Build history of the part. All positions in model axes, mm. A direction names the side the tool comes from. Give positions to 0.01 mm unless a question says otherwise; leave off trailing zeros. Loops run counter-clockwise (first coordinate to the right, second up) from the corner with the lowest first, then second, coordinate; pieces in that order, holes last. Notation, with made-up numbers: M 54,31 L 105,31 A21 cw 105,47 Z; hole C -3.75,-21.75 d2. An arc over 180 degrees is marked long. Put each result on its own line as item: value.
```python
from build123d import *

# Parameters (mm, degrees)
SKETCH1_R               = 5
BOSS_EXTRUDE1_DEPTH     = 2
SKETCH4_R               = 3.9
BOSS_EXTRUDE2_DEPTH     = 16
CUT_EXTRUDE4_DEPTH      = 3
SKETCH3_5_R             = 1.7
CUT_EXTRUDE5_DEPTH      = 3
CUT_EXTRUDE5_DEPTH_BACK = 3.5
SKETCH5_W               = 6.581793069
SKETCH5_H               = 3
CUT_EXTRUDE6_DEPTH      = 6.0375


with BuildPart() as part:
    # Sketch1 → Boss-Extrude1 (new body)
    with BuildSketch(Plane(origin=(0, 0, 0), x_dir=(1, 0, 0), z_dir=(0, 1, 0))):
        Circle(SKETCH1_R)
    extrude(amount=BOSS_EXTRUDE1_DEPTH)

    # Sketch4 → Boss-Extrude2 (add)
    with BuildSketch(Plane(origin=(0, 0, 0), x_dir=(-1, 0, 0), z_dir=(0, -1, 0))):
        Circle(SKETCH4_R)
    extrude(amount=BOSS_EXTRUDE2_DEPTH)

    # Sketch3 → Cut-Extrude4 (cut)
    with BuildSketch(Plane(origin=(0, -13.5, 0), x_dir=(1, 0, 0), z_dir=(0, 1, 0))):
        Polygon((3.225944629, -0.0375), (1.580496362, 2.8125), (-1.710400172, 2.8125), (-3.35584844, -0.0375), (-1.710400172, -2.8875), (1.580496362, -2.8875), align=None)
    extrude(amount=CUT_EXTRUDE4_DEPTH, mode=Mode.SUBTRACT)

    # Sketch3<5> → Cut-Extrude5 (cut, two sides)
    with BuildSketch(Plane(origin=(0, -13.5, 0), x_dir=(1, 0, 0), z_dir=(0, 1, 0))) as cut_extrude5_sk:
        with Locations((-0.064951905, -0.0375)):
            Circle(SKETCH3_5_R)
    extrude(amount=CUT_EXTRUDE5_DEPTH, mode=Mode.SUBTRACT)
    extrude(cut_extrude5_sk.sketch, amount=-CUT_EXTRUDE5_DEPTH_BACK, mode=Mode.SUBTRACT)

    # Sketch5 → Cut-Extrude6 (cut, through all)
    with BuildSketch(Plane.XY.offset(0.0375)):
        with Locations((-0.064951906, -12)):
            Rectangle(SKETCH5_W, SKETCH5_H)
    extrude(amount=-CUT_EXTRUDE6_DEPTH, mode=Mode.SUBTRACT)


solid = part.part
```
Q1. Slice it at A-A (x = 1.25). List the corners of the cut face in (y, z).
Here are the results:
outline: M -16,-3.69 L -13.5,-3.69 L -13.5,-1.04 L -16,-1.04 Z; M -16,1.11 L -13.5,1.11 L -13.5,2.89 L -10.5,2.89 L -10.5,-3.69 L 0,-3.69 L 0,-4.84 L 2,-4.84 L 2,4.84 L 0,4.84 L 0,3.69 L -16,3.69 Z
Q2. Slice it at C-C (y = -11.75). List the corners of the cut face in (x, z).
Here are the results:
outline: M -3.36,-1.99 L -3.36,0.04 L -1.71,2.89 L 1.58,2.89 L 3.23,0.04 L 3.23,-2.19 A3.9 ccw long Z
Q3. Slice it at B-B (z = 2). List the corners of the cut face in (x, y).
Here are the results:
outline: M -4.58,0 L -3.35,0 L -3.35,-16 L 3.35,-16 L 3.35,0 L 4.58,0 L 4.58,2 L -4.58,2 Z; hole M -2.22,-13.5 L 2.09,-13.5 L 2.09,-10.5 L -2.22,-10.5 Z
Q4. Probe line 1 (Y direction, x = 1.5, z = -1.75); line 2 (X direction, y = -14.75, z = 0); line 3 (Y direction, x = -1.25, z = -4.5). List the from-to ranges inside material, lowest first. Write a range as from..to.
Here are the results:
line 1: -16..-13.5, -10.5..2
line 2: -3.9..-1.76, 1.63..3.9
line 3: 0..2
Q5. Slice it at D-D (y = -13.75). List the corners of the cut face in (x, z), and give its area (3 significant figures).
Here are the results:
outline: C 0,0 d7.8; hole C -0.06,0.04 d3.4
area: 38.7 mm²
Q6. Tool access for faces 4 (the flat face through (0, 2, 0)), 5 (the flat face through (2.392, -12.021, 1.482)), 6 (the flat face through (3, 0, 3)): list every direction of +Z, -Z, +X, -X, +Y, -Y with a clear straight run to the whole face (end or side of a thin tool).
Here are the results:
face 4: +Z, -Z, +X, -X, +Y
face 5: -Z
face 6: -Y
Q7. Mould opens along X. For faces 1 (the flat face through (-2, -16, 1)), 2 (the cylindrical face through (-1.08, 0.99, 4.88)), 3 (the flat face through (-2.545, -12.021, 1.443)) say: pulls with the +X half, pulls with the -X half, needs draft (parallel to the pull), parting line crosses it, or undercut.
Here are the results:
face 1: needs draft
face 2: parting line crosses it
face 3: undercut
Q8. Drop flat-ended pins along their axis: pin 1 Ø2 at (x, y) = (1, -3) entering from -Z; pin 2 Ø1 at (y, z) = (-1.5, 0) entering from +X; pin 3 Ø1.6 at (y, z) = (-12.5, -1.5) entering from +X. Give the stop position or say it passes through.
Here are the results:
pin 1: z = -3.9
pin 2: x = 3.9
pin 3: x = 3.84
